```python
from build123d import *

# Parameters (mm, degrees)
WYCI_GNI_CIE1_DEPTH                                 = 30
WYCI_GNI_CIE2_REACH                                 = 332.341
SZKIC3_R                                            = 30
SFAZOWANIE1_SIZE                                    = 2
OTW_R2_OUTLINE_R                                    = 42
OTW_R2_DEPTH                                        = 12.986154641
OTW_R3_OUTLINE_R                                    = 70
OTW_R3_OUTLINE_R_2                                  = 42
OTW_R3_DEPTH                                        = 10
POG_BIENIE_WALCOWE_POD_M8_WKR_T_Z_BEM_W_D           = 9
POG_BIENIE_WALCOWE_POD_M8_WKR_T_Z_BEM_W_CBORE_D     = 15
POG_BIENIE_WALCOWE_POD_M8_WKR_T_Z_BEM_W_CBORE_DEPTH = 8.6


# Read off the part's stored shape, not the designer's step: Otwór2, Otwór3
with BuildPart() as part:
    # Szkic1 → Wyciągnięcie1 (new body)
    with BuildSketch(Plane(origin=(0, 0, 0), x_dir=(1, 0, 0), z_dir=(0, 1, 0))):
        Polygon((-220, -135), (220, -135), (300, -55), (300, 55), (220, 135), (-220, 135), (-300, 55), (-300, -55), align=None)
    extrude(amount=WYCI_GNI_CIE1_DEPTH)

    # Szkic3 → Wyciągnięcie2 (cut, up to next)
    with BuildSketch(Plane(origin=(0, 30, 0), x_dir=(1, 0, 0), z_dir=(0, 1, 0)), mode=Mode.PRIVATE) as wyci_gni_cie2_sk1:
        with Locations(Location((-250, 0, 0), (0, 0, 270))):
            Circle(SZKIC3_R)
    wyci_gni_cie2_tool1 = extrude(wyci_gni_cie2_sk1.sketch, amount=-WYCI_GNI_CIE2_REACH, mode=Mode.PRIVATE) & part.part
    # Szkic3 → Wyciągnięcie2 (cut, up to next)
    with BuildSketch(Plane(origin=(0, 30, 0), x_dir=(1, 0, 0), z_dir=(0, 1, 0)), mode=Mode.PRIVATE) as wyci_gni_cie2_sk2:
        with Locations(Location((250, 0, 0), (0, 0, 270))):
            Circle(SZKIC3_R)
    wyci_gni_cie2_tool2 = extrude(wyci_gni_cie2_sk2.sketch, amount=-WYCI_GNI_CIE2_REACH, mode=Mode.PRIVATE) & part.part
    add(wyci_gni_cie2_tool1.solids().sort_by_distance((-250, 30, 0))[0], mode=Mode.SUBTRACT)
    add(wyci_gni_cie2_tool2.solids().sort_by_distance((250, 30, 0))[0], mode=Mode.SUBTRACT)

    # Sfazowanie1
    sfazowanie1_edges = [part.edges().sort_by_distance(p)[0] for p in [
        (-260, 30, 95),
        (-300, 0, 0),
        (-260, 0, -95),
        (0, 30, 135),
        (260, 30, 95),
        (300, 30, 0),
        (260, 30, -95),
        (-250, 30, -30),
        (-250, 0, -30),
        (0, 30, -135),
        (250, 30, -30),
        (250, 0, -30),
        (-260, 30, -95),
        (-300, 30, 0),
        (0, 0, -135),
        (260, 0, -95),
        (300, 0, 0),
        (260, 0, 95),
        (0, 0, 135),
        (-260, 0, 95),
    ]]
    chamfer(sfazowanie1_edges, length=SFAZOWANIE1_SIZE)

    # Szkic6 → Otwór1 (revolve, cut)
    with BuildSketch(Plane(origin=(0, 30, 0), x_dir=(0, 0, 1), z_dir=(1, 0, 0))):
        Polygon((0, 0), (0, 30), (10, 30), (10, 198.494863687), (45, 0), align=None)
    revolve(axis=Axis((0, 36.445314094, 0), (0, -1, 0)), mode=Mode.SUBTRACT)

    # Otwór2 outline → Otwór2 (cut)
    with BuildSketch(Plane(origin=(0, 0, 0), x_dir=(1, 0, 0), z_dir=(0, 1, 0))):
        Circle(OTW_R2_OUTLINE_R)
    extrude(amount=OTW_R2_DEPTH, mode=Mode.SUBTRACT)

    # Otwór3 outline → Otwór3 (cut)
    with BuildSketch(Plane(origin=(0, 0, 0), x_dir=(1, 0, 0), z_dir=(0, 1, 0))):
        Circle(OTW_R3_OUTLINE_R)
        Circle(OTW_R3_OUTLINE_R_2, mode=Mode.SUBTRACT)
    extrude(amount=OTW_R3_DEPTH, mode=Mode.SUBTRACT)

    # Pogłębienie walcowe pod M8 Wkręt z łbem walcowym z gniazdem sześciokątnym1 (through all)
    with Locations(Plane(origin=(0, 30, 0), x_dir=(1, 0, 0), z_dir=(0, 1, 0))):
        with Locations((-58.015165068, 0), (-29.007582534, 50.242606754), (29.007582534, 50.242606754), (58.015165068, 0), (29.007582534, -50.242606754), (-29.007582534, -50.242606754)):
            CounterBoreHole(POG_BIENIE_WALCOWE_POD_M8_WKR_T_Z_BEM_W_D / 2, POG_BIENIE_WALCOWE_POD_M8_WKR_T_Z_BEM_W_CBORE_D / 2, POG_BIENIE_WALCOWE_POD_M8_WKR_T_Z_BEM_W_CBORE_DEPTH)


solid = part.part
```
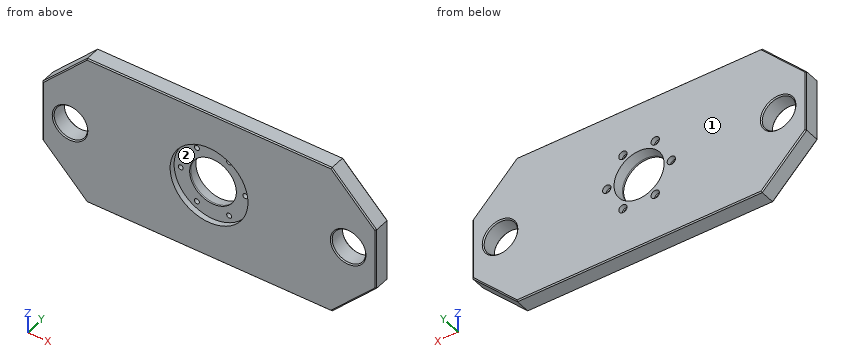
Design review of the part built by this model. Coordinates are the model's own, in mm. Face numbers are marked on the shaded views. Give positions to 0.01 mm unless a question says otherwise; leave off trailing zeros. Order: outer loops, then holes, each group sorted by start corner. A loop starts at its lowest first (then second) coordinate and runs counter-clockwise, first axis right, second up. Notation, with made-up numbers: (-4.75, 78.5) - (40.25, 78.5) arc R8 cw to (40.25, 88.5) - close; hole circle Ø8 at (32, 50.25). An arc over 180 degrees is marked (long way). Use a Markdown table: item, result. Add a question column.
(1) Add section B-B on z = 88.5. Give the boundary of the cut face in (x, y).
(2) Add section C-C on x = -250. Give the boundary of the cut face in (y, z), then the cut area to 3 significant figures.
(3) Add section D-D on z = 18. Give the number of separate pieces and of enclosed holes in the cut face, then the cut area to 3 significant figures.
(4) Wall thickness on probe 1 along Y at (x, z) = (49, 5); probe 2 along Z at (x, y) = (0, 11); probe 3 along X at (y, z) = (21.5, -35.5): over which ranges is each line inside the solid? List them lowest first. Write a range as [from, to].
(5) Add section A-A on x = 0. Give the boundary of the cut face in (y, z), then the cut area to 3 significant figures.
(6) Mouldability with a two-part tool opening along X and no side actions: class the marked faces 1 and 2 as +X half, -X half, draft (parallel to the pull), parting line (faces both ways), or undercut.
(7) Clearance check with flat-ended pins moving along their axes: P1, Ø8, axis at x = -236, y = 9.5, coming from the -Z side; P2, Ø7.5, axis at x = -29, z = 52.5, coming from the +Y side; P3, Ø12, axis at x = 29.01, z = 50.24, coming from the -Y side. State where each tip first meets the part, or that it passes through.
Report:
| question | item | result |
|---|---|---|
| 1 | outline | (-266.5, 2) - (-263.67, 0) - (263.67, 0) - (266.5, 2) - (266.5, 28) - (263.67, 30) - (-263.67, 30) - (-266.5, 28) - close |
| 2 | outline | (0, -102.17) - (2, -105) - (28, -105) - (30, -102.17) - (30, -32) - (28, -30) - (2, -30) - (0, -32) - close; (0, 32) - (2, 30) - (28, 30) - (30, 32) - (30, 102.17) - (28, 105) - (2, 105) - (0, 102.17) - close |
| 2 | area | 4,480 mm² |
| 3 | separate pieces | 4 |
| 3 | enclosed holes | 0 |
| 3 | area | 12,200 mm² |
| 4 | probe 1 | y = [10, 30] |
| 4 | probe 2 | z = [-135, -42], [42, 135] |
| 4 | probe 3 | x = [-300, -25.14], [25.14, 300] |
| 5 | outline | (0, -133) - (2, -135) - (28, -135) - (30, -133) - (30, -45) - (12.99, -42) - (10, -42) - (10, -70) - (0, -70) - close; (0, 70) - (10, 70) - (10, 42) - (12.99, 42) - (30, 45) - (30, 133) - (28, 135) - (2, 135) - (0, 133) - close |
| 5 | area | 4,960 mm² |
| 6 | face 1 | draft |
| 6 | face 2 | undercut |
| 7 | P1 | stops at z = -123 |
| 7 | P2 | stops at y = 21.4 |
| 7 | P3 | stops at y = 10 |
